Verification items for this drawing (mm, ordinates from the low corner). A direction names the side the tool comes from. Round coordinates to 2 decimals unless told otherwise and drop trailing zeros. Order: outer loops, then holes, each group sorted by start corner. A loop starts at its lowest first (then second) coordinate and runs counter-clockwise, first axis right, second up. Notation, with made-up numbers: (4, -9) -> (34, -9) arc R25 cw to (34, 5) -> close; hole circle Ø10 at (41, 83.5). An arc over 180 degrees is marked (long way). Answer in a Markdown table with one row per item. Add a question column.
1. Sectioned sample at B-B, the plane z = 11. Record the boundary of the cut face in (x, y) (1 decimal).
2. Material ranges on L1, parallel to X at y = 2, z = 32.5 (1 decimal); L2, parallel to Z at x = 51, y = 12.5 (1 decimal); L3, parallel to Y at x = 3, z = 5, recorded low to high. Write a range as from..to.
3. Draft check along X on the marked faces 3, 4 and 5. Enter one of: +X half, -X half, draft (parallel to the pull), parting line (faces both ways), or undercut.
4. Access from +Z, -Z, +X, -X, +Y, -Y to the whole of each face (thin tool, end or side, straight path). Record for the marked faces 1 and 2.
5. Depth check by flat-ended pin: P1, Ø1, axis at x = 48.5, y = 22, coming from the +Z side (3 decimals). Enter the tip coordinate at first touch or a pass-through.
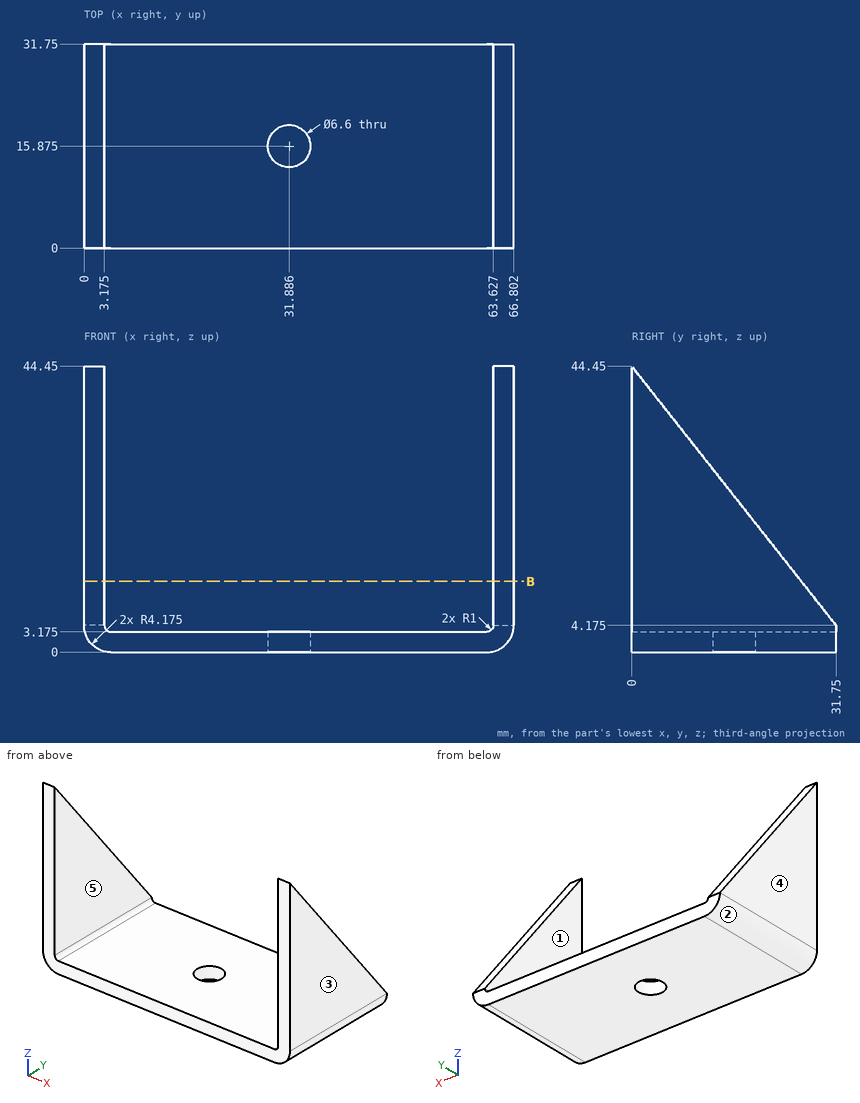
Answer key:
| question | item | result |
|---|---|---|
| 1 | outline | (0, 0) -> (3.2, 0) -> (3.2, 26.4) -> (0, 26.4) -> close; (63.6, 0) -> (66.8, 0) -> (66.8, 26.4) -> (63.6, 26.4) -> close |
| 2 | L1 | x = 0..3.2, 63.6..66.8 |
| 2 | L2 | z = 0..3.2 |
| 2 | L3 | y = 0..31.1 |
| 3 | face 3 | +X half |
| 3 | face 4 | -X half |
| 3 | face 5 | undercut |
| 4 | face 1 | +Z, +Y, -Y |
| 4 | face 2 | -Z, -X, +Y, -Y |
| 5 | P1 | stops at z = 3.175 |
